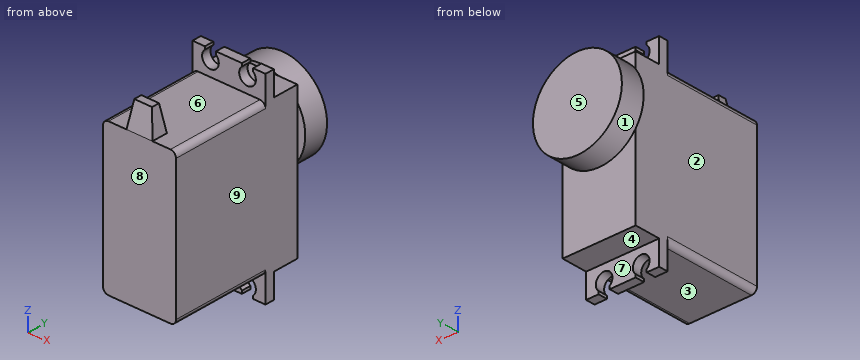
```python
from build123d import *

# Parameters (mm, degrees)
ESQUISSE1_W                         = 40.3
ESQUISSE1_H                         = 36.195
BOSS_EXTRU_1_DEPTH                  = 9.85
ESQUISSE2_W                         = 53.4
ESQUISSE2_H                         = 2.5
BOSS_EXTRU_2_DEPTH                  = 19.7
ESQUISSE3_R                         = 12
BOSS_EXTRU_3_DEPTH                  = 6.5
ESQUISSE5_W                         = 7
ESQUISSE5_H                         = 4.3
BOSS_EXTRU_4_DEPTH                  = 7
BOSS_EXTRU_4_TAPER                  = 9
DIAM_TRE_DU_PER_AGE_4_5_4_5_1_D     = 4.5
DIAM_TRE_DU_PER_AGE_4_5_4_5_1_DEPTH = 3.2
DIAM_TRE_DU_PER_AGE_4_5_4_5_1_TIP   = 1.351936393
ESQUISSE9_W                         = 3
ESQUISSE9_H                         = 0.772949017
ENL_V_MAT_EXTRU_1_DEPTH             = 42.638473795
SYM_TRIE2_COPY_1_SKETCH_W           = 3
SYM_TRIE2_COPY_1_SKETCH_H           = 0.772949017
SYM_TRIE2_COPY_1_DEPTH              = 42.638473795
CONG_1_R                            = 1.5


with BuildPart() as part:
    # Esquisse1 → Boss.-Extru.1 (new, symmetric)
    with BuildSketch(Plane(origin=(0, 0, 0), x_dir=(0, 0, -1), z_dir=(1, 0, 0))):
        Rectangle(ESQUISSE1_W, ESQUISSE1_H)
    extrude(amount=BOSS_EXTRU_1_DEPTH, both=True)

    # Esquisse2 → Boss.-Extru.2 (add)
    with BuildSketch(Plane(origin=(-9.85, 0, 0), x_dir=(0, 0, -1), z_dir=(1, 0, 0))):
        with Locations((0, 9.8525)):
            Rectangle(ESQUISSE2_W, ESQUISSE2_H)
    extrude(amount=BOSS_EXTRU_2_DEPTH)

    # Esquisse3 → Boss.-Extru.3 (add)
    with BuildSketch(Plane(origin=(0, 18.0975, 0), x_dir=(1, 0, 0), z_dir=(0, 1, 0))):
        with Locations(Location((0, -9.15, 0), (0, 0, 34.831699177))):
            Circle(ESQUISSE3_R)
    extrude(amount=BOSS_EXTRU_3_DEPTH)

    # Esquisse5 → Boss.-Extru.4 (add)
    with BuildSketch(Plane.XY.offset(20.15)):
        with Locations((0, -15.9475)):
            Rectangle(ESQUISSE5_W, ESQUISSE5_H)
    extrude(amount=BOSS_EXTRU_4_DEPTH, taper=BOSS_EXTRU_4_TAPER)

    # Diamètre du perçage Ø4.5 (4.5)1
    with Locations(Plane(origin=(0, 11.1025, 0), x_dir=(1, 0, 0), z_dir=(0, 1, 0))):
        with Locations((5, 24.25), (-5, 24.25), (5, -24.25), (-5, -24.25)):
            Hole(DIAM_TRE_DU_PER_AGE_4_5_4_5_1_D / 2, depth=DIAM_TRE_DU_PER_AGE_4_5_4_5_1_DEPTH)
            with Locations((0, 0, -(DIAM_TRE_DU_PER_AGE_4_5_4_5_1_DEPTH + DIAM_TRE_DU_PER_AGE_4_5_4_5_1_TIP / 2))):  # 118° drill point
                Cone(0, DIAM_TRE_DU_PER_AGE_4_5_4_5_1_D / 2, DIAM_TRE_DU_PER_AGE_4_5_4_5_1_TIP, mode=Mode.SUBTRACT)

    # Esquisse9 → Enlèv. mat.-Extru.1 (cut, through all)
    with BuildSketch(Plane(origin=(0, 11.1025, 0), x_dir=(1, 0, 0), z_dir=(0, 1, 0))):
        with Locations((-5, 26.313525492)):
            Rectangle(ESQUISSE9_W, ESQUISSE9_H)
    enl_v_mat_extru_1 = extrude(amount=-ENL_V_MAT_EXTRU_1_DEPTH, mode=Mode.SUBTRACT)

    # Symétrie1: Enlèv. mat.-Extru.1 across plane
    add(enl_v_mat_extru_1.mirror(Plane(origin=(0, 0, 0), x_dir=(0, 0, 1), z_dir=(1, 0, 0))), mode=Mode.SUBTRACT)

    # Symétrie2: Enlèv. mat.-Extru.1 across plane
    add(enl_v_mat_extru_1.mirror(Plane.XY), mode=Mode.SUBTRACT)

    # Symétrie2 copy 1 sketch → Symétrie2 copy 1 (cut, through all)
    with BuildSketch(Plane(origin=(0, 11.1025, 0), x_dir=(-1, 0, 0), z_dir=(0, 1, 0))):
        with Locations((-5, 26.313525492)):
            Rectangle(SYM_TRIE2_COPY_1_SKETCH_W, SYM_TRIE2_COPY_1_SKETCH_H)
    extrude(amount=-SYM_TRIE2_COPY_1_DEPTH, mode=Mode.SUBTRACT)

    # Congé1
    cong_1_edges = [part.edges().sort_by_distance(p)[0] for p in [
        (-9.85, -4.7475, 20.15),
        (9.85, -4.7475, 20.15),
        (9.85, -4.7475, -20.15),
        (-9.85, -4.7475, -20.15),
    ]]
    fillet(cong_1_edges, radius=CONG_1_R)


solid = part.part
```
The listing builds one solid part. Answer for the finished solid, in the listing's coordinates (mm). Face numbers are marked on the shaded views. A direction names the side the tool comes from. Give positions to 0.01 mm unless a question says otherwise; leave off trailing zeros. Loops run counter-clockwise (first coordinate to the right, second up) from the corner with the lowest first, then second, coordinate; pieces in that order, holes last. Notation, with made-up numbers: (55.25, -3) - (84.25, -3) arc R13 ccw to (84.25, 21) - close; hole circle Ø11 at (52, 46.5). An arc over 180 degrees is marked (long way). Answer as CSV lines item,"result". Start each with the question number.
Item 1: A cutting plane is placed at B-B on y = -8.5. Determine the outline of the cut face in (x, z).
Item 2: Find the intervals of material crossed by line 1 (X direction, y = 9.2, z = 24.25); line 2 (Y direction, x = -7.75, z = 24); line 3 (Y direction, x = -5.25, z = -11), in increasing order. Write a range as from..to.
Item 3: For the marked faces 1, 2, 3, 4 and 5, determine the directions among +Z, -Z, +X, -X, +Y, -Y from which every point of the face is accessible in a straight line to the end or side of a thin tool.
Item 4: A cutting plane is placed at D-D on x = 0. Determine the outline of the cut face in (y, z), then the cut area to 3 significant figures.
Item 5: A cutting plane is placed at A-A on z = -24.25. Determine the outline of the cut face in (x, y), then the cut area to 4 significant figures.
Item 6: A cutting plane is placed at C-C on z = 9.15. Determine the outline of the cut face in (x, y).
Item 7: Each of these flat-tipped pins is pushed along its axis until it touches: pin 1 (10 mm diameter, centred on x = 0.5, z = -10.5, fed in from +Y); pin 2 (2 mm diameter, centred on x = 3.5, y = 16, fed in from -Z); pin 3 (4 mm diameter, centred on y = 2, z = 9.5, fed in from -X). Where does it stop, or does it pass through?
Item 8: The mould has two halves that part along Y. Classify the marked faces 6, 7, 8 and 9: +Y half, -Y half, draft (parallel to the pull), parting line (faces both ways), or undercut.
Found:
1,outline,"(-9.85, -18.65) arc R1.5 ccw to (-8.35, -20.15) - (8.35, -20.15) arc R1.5 ccw to (9.85, -18.65) - (9.85, 18.65) arc R1.5 ccw to (8.35, 20.15) - (-8.35, 20.15) arc R1.5 ccw to (-9.85, 18.65) - close"
2,line 1,"x = -9.85..-7.25, -2.75..2.75, 7.25..9.85"
2,line 2,"y = 8.6..11.1"
2,line 3,"y = -18.1..18.1"
3,face 1,"+Y"
3,face 2,"+Z, -Z, -X, -Y"
3,face 3,"-Z, +X, -X, -Y"
3,face 4,"-Z, +X, -X, +Y"
3,face 5,"+Z, -Z, +X, -X, +Y"
4,outline,"(-18.1, -20.15) - (8.6, -20.15) - (8.6, -26.7) - (11.1, -26.7) - (11.1, -20.15) - (18.1, -20.15) - (18.1, -2.85) - (24.6, -2.85) - (24.6, 21.15) - (18.1, 21.15) - (18.1, 20.15) - (11.1, 20.15) - (11.1, 26.7) - (8.6, 26.7) - (8.6, 20.15) - (-13.8, 20.15) - (-14.91, 27.15) - (-16.99, 27.15) - (-18.1, 20.15) - close"
4,area,"1,670 mm^2"
5,outline,"(-9.85, 8.6) - (-7.25, 8.6) - (-7.25, 11.1) - (-9.85, 11.1) - close; (-2.75, 8.6) - (2.75, 8.6) - (2.75, 11.1) - (-2.75, 11.1) - close; (7.25, 8.6) - (9.85, 8.6) - (9.85, 11.1) - (7.25, 11.1) - close"
5,area,"26.75 mm^2"
6,outline,"(-12, 18.1) - (-9.85, 18.1) - (-9.85, -18.1) - (9.85, -18.1) - (9.85, 18.1) - (12, 18.1) - (12, 24.6) - (-12, 24.6) - close"
7,pin 1,"stops at y = 18.1"
7,pin 2,"stops at z = -20.15"
7,pin 3,"stops at x = -9.85"
8,face 6,"undercut"
8,face 7,"+Y half"
8,face 8,"-Y half"
8,face 9,"draft"
